Work out the finished part from the listing and answer in its coordinate system (mm). A direction names the side the tool comes from. Round coordinates to 2 decimals unless told otherwise and drop trailing zeros. Order: outer loops, then holes, each group sorted by start corner. A loop starts at its lowest first (then second) coordinate and runs counter-clockwise, first axis right, second up. Notation, with made-up numbers: (17.5, 33) - (33.5, 33) arc R20 ccw to (33.5, 40) - close; hole circle Ø3 at (23.5, -21). An arc over 180 degrees is marked (long way). Use one line per item in the form item = value. Start each with the question number.
Q1. Find the intervals of material crossed by line 1 (Z direction, x = -195, y = -15); line 2 (Y direction, x = -110.5, z = 8.25); line 3 (Y direction, x = 171, z = -12.85), in increasing order. Write a range as [from, to].
Q2. The part is cut by section A-A on y = 5. Determine the outline of the cut face in (x, z), plus the area to 3 significant figures.
Q3. The part is cut by section B-B on x = -90.5. Determine the outline of the cut face in (y, z), plus the area to 3 significant figures.
Q4. For a pull along Z with two mould halves and no side action, classify faces 3 (the flat face through (-19, 0, 12)), 4 (the flat face through (181, -2, -12.2)), 5 (the flat face through (-19, 0, 15)) as +Z half, -Z half, draft (parallel to the pull), parting line (faces both ways), or undercut.
Q5. Which of the six approach directions +Z, -Z, +X, -X, +Y, -Y give full straight-line access (tool end or side, diameter ignored) to faces 1 (the flat face through (-19, 22, 0)), 2 (the flat face through (-19, 25, 0))?
Q6. Given P1, Ø4, axis at x = -171, y = -16, coming from the -Z side, flat-ended and moving along its own axis, determine where the tip first touches the part or whether it passes through.
from build123d import *

# Parameters (mm, degrees)
F0_W     = 50
F0_H     = 30
F0_W_2   = 44
F0_H_2   = 24
F1_DEPTH = 181
F2_R     = 1.5
F3_R     = 4.5
F4_R     = 3.25
F5_DEPTH = 35
F6_SIZE  = 0.5
F7_DEPTH = 43


with BuildPart() as f1:
    # F0 (on Right) → F1 (new body, symmetric)
    with BuildSketch(Plane.YZ):
        Rectangle(F0_W, F0_H)
        Rectangle(F0_W_2, F0_H_2, mode=Mode.SUBTRACT)
    extrude(amount=F1_DEPTH, both=True)

    # F2
    f2_edges = [f1.edges().sort_by_distance(p)[0] for p in [
        (0, -22, -12),
        (0, -22, 12),
        (0, 22, -12),
        (0, 22, 12),
    ]]
    fillet(f2_edges, radius=F2_R)

    # F3
    f3_edges = [f1.edges().sort_by_distance(p)[0] for p in [
        (0, -25, 15),
        (0, -25, -15),
        (0, 25, -15),
        (0, 25, 15),
    ]]
    fillet(f3_edges, radius=F3_R)

    # F4 (on face) → F5 (cut)
    with BuildSketch(Plane.XY.offset(15)):
        with Locations((-171, 16)):
            Circle(F4_R)
        with Locations((-171, -16)):
            Circle(F4_R)
        with Locations((171, -16)):
            Circle(F4_R)
        with Locations((171, 16)):
            Circle(F4_R)
    extrude(amount=-F5_DEPTH, mode=Mode.SUBTRACT)

    # F6
    f6_edges = [f1.edges().sort_by_distance(p)[0] for p in [
        (-174.25, -16, 15),
        (-174.25, 16, 15),
        (167.75, -16, 15),
        (167.75, 16, 15),
        (167.75, 16, -15),
        (167.75, -16, -15),
        (-174.25, 16, -15),
        (-174.25, -16, -15),
    ]]
    chamfer(f6_edges, length=F6_SIZE)

    # F7 (add): a face of the model
    f7_faces = [f1.faces().sort_by_distance(p)[0] for p in [
        (-181, -24.4169048105, 0),
    ]]
    extrude(f7_faces, amount=F7_DEPTH)


solid = f1.part
Found:
q1.line_1 = [-15, -12], [12, 15]
q1.line_2 = [-25, -22], [22, 25]
q1.line_3 = [-24.34, -19.25], [-12.75, 12.75], [19.25, 24.34]
q2.outline = (-224, -15) - (181, -15) - (181, -12) - (-224, -12) - close; (-224, 12) - (181, 12) - (181, 15) - (-224, 15) - close
q2.area = 2,430 mm²
q3.outline = (-25, -10.5) arc R4.5 ccw to (-20.5, -15) - (20.5, -15) arc R4.5 ccw to (25, -10.5) - (25, 10.5) arc R4.5 ccw to (20.5, 15) - (-20.5, 15) arc R4.5 ccw to (-25, 10.5) - close; hole (-22, -10.5) arc R1.5 ccw to (-20.5, -12) - (20.5, -12) arc R1.5 ccw to (22, -10.5) - (22, 10.5) arc R1.5 ccw to (20.5, 12) - (-20.5, 12) arc R1.5 ccw to (-22, 10.5) - close
q3.area = 429 mm²
q4.face_3 = undercut
q4.face_4 = draft
q4.face_5 = +Z half
q5.face_1 = +X, -X
q5.face_2 = +Z, -Z, +X, -X, +Y
q6.P1 = through
